Autodesk Inventor part; units mm, degrees
ref_plane "YZ Plane" through (0, 0, 0) normal (1, 0, 0) x (0, 1, 0)
ref_plane "XZ Plane" through (0, 0, 0) normal (0, 1, 0) x (-1, 0, 0)
ref_plane "XY Plane" through (0, 0, 0) normal (0, 0, 1) x (1, 0, 0)
sketch "Sketch1" plane through (0, 0, 0) normal (0, 0, 1) x (1, 0, 0)
  line L0 (0, 0) -> (9.5, 0)
  line L1 (9.5, 0) -> (9.5, 9.5)
  line L2 (9.5, 9.5) -> (0, 9.5)
  line L3 (0, 9.5) -> (0, 0)
  dimension "d0" = 9.5
  dimension "d1" = 9.5
extrude "Extrusion1" add sketch "Sketch1" along normal blind 24
sketch "Sketch2" plane through (0, 9.5, 0) normal (0, 1, 0) x (1, 0, 0)
  line L0 (0, -24) -> (9.5, -24)
  line L1 (2.25, -24) -> (7.25, -24)
  line L2 (7.25, -24) -> (7.25, -9.5)
  line L3 (7.25, -9.5) -> (2.25, -9.5)
  line L4 (2.25, -9.5) -> (2.25, -24)
  line L5 (0, 0) -> (0, -24)
  dimension "d4" = 14.5
  dimension "d5" = 5
  dimension "d6" = 2.25
extrude "Extrusion2" cut sketch "Sketch2" against normal up to next
sketch "Sketch3" plane through (9.5, 0, 0) normal (1, 0, 0) x (0, 0, -1)
  circle A0 centre (-19, 4.75) radius 2.5
  line L0 (-24, 0) -> (-24, 9.5)
  line L1 (0, 9.5) -> (-24, 9.5)
  point P0 (0, 0)
  dimension "d9" = 5
  dimension "d10" = 5
  dimension "d11" = 4.75
extrude "Extrusion3" cut sketch "Sketch3" against normal through all
sketch "Sketch4" plane through (2.25, 9.5, 9.5) normal (0, 0, 1) x (1, 0, 0)
  circle A0 centre (2.5, -4.75) radius 2
  line L0 (0, 0) -> (5, 0)
  line L1 (0, -9.5) -> (0, 0)
  point P0 (-2.25, -9.5)
  dimension "d14" = 4
  dimension "d15" = 4.75
  dimension "d16" = 2.5
extrude "Extrusion4" cut sketch "Sketch4" against normal up to next
properties part number "piston_rod_connector" material "Steel, Non-Alloy"
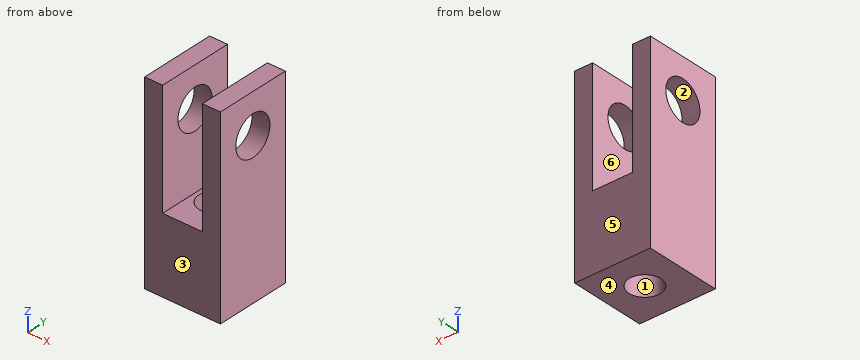
Read the model definition and answer for the solid it produces. Units are mm, in the model's axes. Face numbers are marked on the shaded views. A direction names the side the tool comes from. Give positions to 0.01 mm unless a question says otherwise; leave off trailing zeros. Write each loop counter-clockwise with the first axis right and the second up, starting at its lowest first coordinate (ties: lowest second). Pieces come first, ordered by that corner, then holes. Notation, with made-up numbers: (0, 78.5) - (36, 78.5) arc R18 ccw to (36, 104.5) - close; hole circle Ø9 at (31, 50.25). An arc over 180 degrees is marked (long way). Answer in a Markdown table with one row per item. Add a question column.
Item 1: Section B-B, the plane y = 4.75 is taken. Write down the section's boundary in (x, z).
Item 2: Find the intervals of material crossed by L1, parallel to Y at x = 7.85, z = 19; L2, parallel to Y at x = 6, z = 9.25, in increasing order.
Item 3: Determine the mould class of the marked faces 1, 2, 3 and 4 for opening direction Y: pulls with the +Y half, pulls with the -Y half, needs draft (parallel to the pull), parting line crosses it, or undercut.
Item 4: A flat-ended cylindrical pin translates along its axis: P1, Ø4, axis at x = 4.5, y = 6, coming from the +Z side. Find the tip coordinate at first contact, or state that the pin passes through.
Item 5: Section A-A, the plane x = 4.75 is taken. Write down the section's boundary in (y, z).
Item 6: Section C-C, the plane z = 19 is taken. Write down the section's boundary in (x, y), and give its area (4 significant figures).
Item 7: A tool of negligible diameter and unlimited length cuts with its end or side. For the marked faces 5 and 6, from which of +Z, -Z, +X, -X, +Y, -Y can it reach the whole face along a straight path? Write none if from no direction.
Item 8: Section D-D, the plane z = 9.25 is taken. Write down the section's boundary in (x, y), and give its area (3 significant figures).
Recorded:
| question | item | result |
|---|---|---|
| 1 | outline | (0, 0) - (2.75, 0) - (2.75, 9.5) - (2.25, 9.5) - (2.25, 16.5) - (0, 16.5) - close; (0, 21.5) - (2.25, 21.5) - (2.25, 24) - (0, 24) - close; (6.75, 0) - (9.5, 0) - (9.5, 16.5) - (7.25, 16.5) - (7.25, 9.5) - (6.75, 9.5) - close; (7.25, 21.5) - (9.5, 21.5) - (9.5, 24) - (7.25, 24) - close |
| 2 | L1 | y = 0 to 2.25, 7.25 to 9.5 |
| 2 | L2 | y = 0 to 3.19, 6.31 to 9.5 |
| 3 | face 1 | undercut |
| 3 | face 2 | undercut |
| 3 | face 3 | pulls with the -Y half |
| 3 | face 4 | needs draft |
| 4 | P1 | stops at z = 9.5 |
| 5 | outline | (0, 0) - (2.75, 0) - (2.75, 9.5) - (0, 9.5) - close; (6.75, 0) - (9.5, 0) - (9.5, 9.5) - (6.75, 9.5) - close |
| 6 | outline | (0, 0) - (2.25, 0) - (2.25, 2.25) - (0, 2.25) - close; (0, 7.25) - (2.25, 7.25) - (2.25, 9.5) - (0, 9.5) - close; (7.25, 0) - (9.5, 0) - (9.5, 2.25) - (7.25, 2.25) - close; (7.25, 7.25) - (9.5, 7.25) - (9.5, 9.5) - (7.25, 9.5) - close |
| 6 | area | 20.25 mm2 |
| 7 | face 5 | +Z, -Z, +X, -X, +Y |
| 7 | face 6 | +Z, +Y, -Y |
| 8 | outline | (0, 0) - (9.5, 0) - (9.5, 9.5) - (0, 9.5) - close; hole circle Ø4 at (4.75, 4.75) |
| 8 | area | 77.7 mm2 |
